CAD build for the part. Positions are in the model's coordinates, mm. A direction names the side the tool comes from. Coordinates: 2 decimals unless noted, no trailing zeros. One line per item, written item: value.
from build123d import *

# Parameters (mm, degrees)
SKETCH1_R           = 2.5019
BOSS_EXTRUDE1_DEPTH = 5.08
FILLET1_R           = 2.54
FILLET2_R           = 2.54
SKETCH2_R           = 1.75
CUT_EXTRUDE1_DEPTH  = 186.472184555


with BuildPart() as part:
    # Sketch1 → Boss-Extrude1 (new body)
    with BuildSketch(Plane.XY):
        with BuildLine():
            Line((27.708128771, -12.7), (124.691871229, -12.7))
            ThreePointArc((124.691871229, -12.7), (182.88, 0), (124.691871229, 12.7))
            Line((124.691871229, 12.7), (27.708128771, 12.7))
            ThreePointArc((27.708128771, 12.7), (-30.48, 0), (27.708128771, -12.7))
        make_face()
        with Locations((152.4, 0)):
            Circle(SKETCH1_R, mode=Mode.SUBTRACT)
        with BuildLine():
            Line((-1.67829283, 1.855488288), (-1.67829283, -1.855488288))
            ThreePointArc((-1.67829283, -1.855488288), (2.5019, 0), (-1.67829283, 1.855488288))
        make_face(mode=Mode.SUBTRACT)
    extrude(amount=BOSS_EXTRUDE1_DEPTH)

    # Fillet1
    fillet1_edges = [part.edges().sort_by_distance(p)[0] for p in [
        (-30.48, 0, 5.08),
        (76.2, -12.7, 5.08),
        (182.88, 0, 5.08),
        (76.2, 12.7, 5.08),
    ]]
    fillet(fillet1_edges, radius=FILLET1_R)

    # Fillet2
    fillet2_edges = [part.edges().sort_by_distance(p)[0] for p in [
        (76.2, -12.7, 0),
        (-30.48, 0, 0),
        (76.2, 12.7, 0),
        (182.88, 0, 0),
    ]]
    fillet(fillet2_edges, radius=FILLET2_R - 0.0001)  # a hair under: the kernel refuses the full size

    # Sketch2 → Cut-Extrude1 (cut, through all)
    with BuildSketch(Plane.XY.offset(5.08)):
        with Locations((21.920310217, 0)):
            Circle(SKETCH2_R)
        with Locations((0, -21.920310217)):
            Circle(SKETCH2_R)
        with Locations((-21.920310217, 0)):
            Circle(SKETCH2_R)
        with Locations((0, 21.920310217)):
            Circle(SKETCH2_R)
    cut_extrude1 = extrude(amount=-CUT_EXTRUDE1_DEPTH, mode=Mode.SUBTRACT)

    # Mirror1: Cut-Extrude1 across plane
    add(cut_extrude1.mirror(Plane(origin=(76.2, 0, 0), x_dir=(0, 0, 1), z_dir=(1, 0, 0))), mode=Mode.SUBTRACT)


solid = part.part
Q1. Slice it at B-B (z = 3.7). Give the number of separate pieces and of enclosed holes in the cut face, plus the area to 3 significant figures.
Recorded:
separate pieces: 1
enclosed holes: 10
area: 7,940 mm^2
Q2. Mould opens along Y. For faces 3 (the face through (2.5, -0.1, 2.5)), 4 (the face through (75, 0, 0)), 5 (the face through (-0.228, 23.655, 2.576)) say: released by +Y, released by -Y, zero draft, split by the parting line, or undercut.
Recorded:
face 3: undercut
face 4: zero draft
face 5: undercut
Q3. Pin check, flat tips, straight feed: pin 1 Ø2 at (y, z) = (24.5, 2.5) entering from +X; pin 2 Ø1 at (x, z) = (63, 1.5) entering from -Y; pin 3 Ø2 at (x, z) = (101.5, 4.5) entering from +Y. Stop position of each tip, or through.
Recorded:
pin 1: stops at x = 171.81
pin 2: stops at y = -12.64
pin 3: stops at y = 12.51
Q4. Drill centre lines: line 1 along Y through (x, z) = (152.4, 2.35); line 2 along X through (y, z) = (13.5, 3.3); line 3 along X through (y, z) = (26.5, 2.35). Where is each one in solid material? Low to high.
Recorded:
line 1: y = -30.47 to -23.67, -20.17 to -2.5, 2.5 to 20.17, 23.67 to 30.47
line 2: x = -27.2 to 27.2, 125.2 to 179.6
line 3: x = -15.04 to 15.04, 137.36 to 167.44
Q5. Which spindle directions (+Z, -Z, +X, -X, +Y, -Y) get a long thin tool onto all of the face, cutting with end or side? Do faces 1 (the face through (75, 0, 5.08)), 2 (the face through (-1.678, 0, 3)). Say none if no direction does.
Recorded:
face 1: +Z, +X, -X, +Y, -Y
face 2: +Z, -Z
